Design review of the part built by this model. Coordinates are the model's own, in mm. Coordinates: 2 decimals unless noted, no trailing zeros. Write each loop counter-clockwise with the first axis right and the second up, starting at its lowest first coordinate (ties: lowest second). Pieces come first, ordered by that corner, then holes. Notation, with made-up numbers: M 7.5,57 L 47.5,57 A24 ccw 47.5,69 Z; hole C 42,14 d8. An arc over 180 degrees is marked long. Write item = value, one per line.
```python
from build123d import *

# Parameters (mm, degrees)
EXTRUDE1_DEPTH        = 6.4
M8X1_0_TAPPED_HOLE1_D = 7


with BuildPart() as part:
    # Sketch1 → Extrude1 (new body)
    with BuildSketch(Plane.XY):
        Polygon((7.390083446, 0), (3.695041723, 6.4), (-3.695041723, 6.4), (-7.390083446, 0), (-3.695041723, -6.4), (3.695041723, -6.4), align=None)
    extrude(amount=EXTRUDE1_DEPTH)

    # M8x1.0 Tapped Hole1 (through all)
    with Locations(Plane.XY.offset(6.4)):
        with Locations((0, 0)):
            Hole(M8X1_0_TAPPED_HOLE1_D / 2)


solid = part.part
```
Q1. Consider section D-D, the plane y = -4.5. State the section outline as (x, z) points.
Check result:
outline = M -4.79,0 L 4.79,0 L 4.79,6.4 L -4.79,6.4 Z
Q2. Consider section C-C, the plane y = -0.5. State the section outline as (x, z) points, and give its area (3 significant figures).
Check result:
outline = M -7.1,0 L -3.46,0 L -3.46,6.4 L -7.1,6.4 Z; M 3.46,0 L 7.1,0 L 7.1,6.4 L 3.46,6.4 Z
area = 46.6 mm²
Q3. Consider section A-A, the plane x = 0. State the section outline as (y, z) points.
Check result:
outline = M -6.4,0 L -3.5,0 L -3.5,6.4 L -6.4,6.4 Z; M 3.5,0 L 6.4,0 L 6.4,6.4 L 3.5,6.4 Z
Q4. The part is to be moulded in two halves that separate along Y. For faces 1 (the cylindrical face through (-3.233, -1.341, 3.155)), 2 (the flat face through (-5.52, 3.24, 3.16)), 3 (the flat face through (3, 3, 6.4)), say which applies: +Y half, -Y half, draft (parallel to the pull), parting line (faces both ways), or undercut.
Check result:
face_1 = undercut
face_2 = +Y half
face_3 = draft
Q5. Wall thickness on line 1 (Y direction, x = 0, z = 4); line 2 (X direction, y = -3, z = 2.5); line 3 (Y direction, x = -1, z = 6.25): over which ranges is each line inside the solid? List them lowest first.
Check result:
line_1 = -6.4 to -3.5, 3.5 to 6.4
line_2 = -5.66 to -1.8, 1.8 to 5.66
line_3 = -6.4 to -3.35, 3.35 to 6.4
Q6. Consider section B-B, the plane z = 5.5. State the section outline as (x, y) points.
Check result:
outline = M -7.39,0 L -3.7,-6.4 L 3.7,-6.4 L 7.39,0 L 3.7,6.4 L -3.7,6.4 Z; hole C 0,0 d7
